For this review, take the finished solid that the model builds, in its own axes (mm). A direction names the side the tool comes from. Coordinates: 2 decimals unless noted, no trailing zeros. Write each loop counter-clockwise with the first axis right and the second up, starting at its lowest first coordinate (ties: lowest second). Pieces come first, ordered by that corner, then holes.
1) To check wall thickness, follow line 1 along Y through (x, z) = (-70.5, 8.9); line 2 along Y through (x, z) = (70.5, 4); line 3 along X through (y, z) = (-6, 2.5) (3 decimals). State the ranges of each line that lie inside material, in increasing order.
2) Insertion check: P1, Ø6.5, axis at x = 71.5, y = 67.5, coming from the -Z side; P2, Ø6.5, axis at x = -67.5, y = 66.5, coming from the -Z side; P3, Ø22, axis at x = -32.4, y = -6, coming from the +Z side. Each pin has a flat end and moves straight along its axis. Give the tip position at first contact, or say it passes through.
3) We need section B-B on y = -108. Write out the cut boundary in (x, z) (3 decimals).
4) We need section A-A on z = 3.75. Write out the cut boundary in (x, y) (3 decimals).
5) For faces 4 (the face through (-22.135, -5.548, 3.944)), 5 (the face through (-76.935, -132.852, 10.497)), 6 (the face through (90.5, -2, 6)), list the 3-axis set-ups (+Z, -Z, +X, -X, +Y, -Y) from which the entire face can be reached by the end or side of a thin tool; tool diameter is ignored.
6) Mouldability with a two-part tool opening along X and no side actions: class faces 1 (the face through (-88, 34, 12)), 2 (the face through (-90.5, -2, 6)), 3 (the face through (-35.5, -1.1, 9)) as pulls with the +X half, pulls with the -X half, needs draft (parallel to the pull), parting line crosses it, or undercut.
7) We need section C-C on x = -70.5. Write out the cut boundary in (y, z) (3 decimals).
from build123d import *

# Parameters (mm, degrees)
ESBO_O1_W                                           = 181
ESBO_O1_H                                           = 296
RESSALTO_EXTRUS_O1_DEPTH                            = 12
FILETE1_R                                           = 2
FILETE2_R                                           = 2
ESBO_O4_W                                           = 3.53
ESBO_O4_H                                           = 3.53
REBAIXO_PARA_PARAFUSO_COM_CABE_A_PANELA_D           = 7
REBAIXO_PARA_PARAFUSO_COM_CABE_A_PANELA_CBORE_D     = 13
REBAIXO_PARA_PARAFUSO_COM_CABE_A_PANELA_CBORE_DEPTH = 8
CORTE_EXTRUS_O1_REACH                               = 175.891
ESBO_O9_R                                           = 5.8
ESBO_O10_R                                          = 10.275
CORTE_EXTRUS_O2_DEPTH                               = 8
ESBO_O11_R                                          = 13.75
CORTE_EXTRUS_O3_DEPTH                               = 2
CORTE_EXTRUS_O4_DEPTH                               = 1.4
CORTE_EXTRUS_O5_DEPTH                               = 1.4


with BuildPart() as part:
    # Esboço1 → Ressalto-extrusão1 (new body)
    with BuildSketch(Plane.XY):
        Rectangle(ESBO_O1_W, ESBO_O1_H)
    extrude(amount=RESSALTO_EXTRUS_O1_DEPTH)

    # Filete1
    filete1_edges = [part.edges().sort_by_distance(p)[0] for p in [
        (-90.5, 148, 6),
    ]]
    fillet(filete1_edges, radius=FILETE1_R)

    # Filete2
    filete2_edges = [part.edges().sort_by_distance(p)[0] for p in [
        (90.5, -148, 6),
        (-90.5, -148, 6),
        (90.5, 148, 6),
    ]]
    fillet(filete2_edges, radius=FILETE2_R)

    # Varredura de corte1: sweep along a path in Esboço2
    with BuildLine(Plane.XY.offset(12)) as varredura_de_corte1_path:
        Line((-63.9, -140.1), (64.1, -140.1))
        ThreePointArc((64.1, -140.1), (78.242135624, -134.242135624), (84.1, -120.1))
        Line((84.1, -120.1), (84.1, 119.9))
        ThreePointArc((84.1, 119.9), (78.242135624, 134.042135624), (64.1, 139.9))
        Line((64.1, 139.9), (-63.9, 139.9))
        ThreePointArc((-63.9, 139.9), (-78.042135624, 134.042135624), (-83.9, 119.9))
        Line((-83.9, 119.9), (-83.9, -120.1))
        ThreePointArc((-83.9, -120.1), (-78.042135624, -134.242135624), (-63.9, -140.1))
    # Esboço4 → Varredura de corte1 (sweep, cut)
    with BuildSketch(Plane(origin=(0, 0, 0), x_dir=(1, 0, 0), z_dir=(0, 1, 0))):
        with Locations((-83.9, -10.8)):
            Rectangle(ESBO_O4_W, ESBO_O4_H)
    sweep(path=varredura_de_corte1_path.line, mode=Mode.SUBTRACT)

    # Rebaixo para parafuso com cabeça panela de M61 (through all)
    with Locations(Plane(origin=(0, 0, 0), x_dir=(-1, 0, 0), z_dir=(0, 0, -1))):
        with Locations((-70.5, 68), (70.5, 68), (70.5, -108), (-70.5, -108)):
            CounterBoreHole(REBAIXO_PARA_PARAFUSO_COM_CABE_A_PANELA_D / 2, REBAIXO_PARA_PARAFUSO_COM_CABE_A_PANELA_CBORE_D / 2, REBAIXO_PARA_PARAFUSO_COM_CABE_A_PANELA_CBORE_DEPTH)

    # Esboço9 → Corte-extrusão1 (cut, up to next)
    with BuildSketch(Plane(origin=(0, 0, 0), x_dir=(-1, 0, 0), z_dir=(0, 0, -1)), mode=Mode.PRIVATE) as corte_extrus_o1_sk1:
        with Locations((32.4, -6)):
            Circle(ESBO_O9_R)
    corte_extrus_o1_tool1 = extrude(corte_extrus_o1_sk1.sketch, amount=-CORTE_EXTRUS_O1_REACH, mode=Mode.PRIVATE) & part.part
    # Esboço9 → Corte-extrusão1 (cut, up to next)
    with BuildSketch(Plane(origin=(0, 0, 0), x_dir=(-1, 0, 0), z_dir=(0, 0, -1)), mode=Mode.PRIVATE) as corte_extrus_o1_sk2:
        with Locations((-32.4, 8.8)):
            Circle(ESBO_O9_R)
    corte_extrus_o1_tool2 = extrude(corte_extrus_o1_sk2.sketch, amount=-CORTE_EXTRUS_O1_REACH, mode=Mode.PRIVATE) & part.part
    add(corte_extrus_o1_tool1.solids().sort_by_distance((-32.4, -6, 0))[0], mode=Mode.SUBTRACT)
    add(corte_extrus_o1_tool2.solids().sort_by_distance((32.4, 8.8, 0))[0], mode=Mode.SUBTRACT)

    # Esboço10 → Corte-extrusão2 (cut)
    with BuildSketch(Plane(origin=(0, 0, 0), x_dir=(-1, 0, 0), z_dir=(0, 0, -1))):
        with Locations((32.4, -6)):
            Circle(ESBO_O10_R)
        with Locations((-32.4, 8.8)):
            Circle(ESBO_O10_R)
    extrude(amount=-CORTE_EXTRUS_O2_DEPTH, mode=Mode.SUBTRACT)

    # Esboço11 → Corte-extrusão3 (cut)
    with BuildSketch(Plane.XY.offset(12)):
        with Locations((32.4, 8.8)):
            Circle(ESBO_O11_R)
        with Locations((-32.4, -6)):
            Circle(ESBO_O11_R)
    extrude(amount=-CORTE_EXTRUS_O3_DEPTH, mode=Mode.SUBTRACT)

    # Esboço12 → Corte-extrusão4 (cut)
    with BuildSketch(Plane(origin=(0, 0, 0), x_dir=(-1, 0, 0), z_dir=(0, 0, -1))):
        with BuildLine():
            Line((-33.4, 19.075), (-33.4, 25.075))
            ThreePointArc((-33.4, 25.075), (-32.4, 26.075), (-31.4, 25.075))
            Line((-31.4, 25.075), (-31.4, 19.075))
            ThreePointArc((-31.4, 19.075), (-32.4, 18.075), (-33.4, 19.075))
        make_face()
    extrude(amount=-CORTE_EXTRUS_O4_DEPTH, mode=Mode.SUBTRACT)

    # Esboço13 → Corte-extrusão5 (cut)
    with BuildSketch(Plane(origin=(0, 0, 0), x_dir=(-1, 0, 0), z_dir=(0, 0, -1))):
        with BuildLine():
            Line((31.4, 4.275), (31.4, 9.275))
            ThreePointArc((31.4, 9.275), (32.4, 10.275), (33.4, 9.275))
            Line((33.4, 9.275), (33.4, 4.275))
            ThreePointArc((33.4, 4.275), (32.4, 3.275), (31.4, 4.275))
        make_face()
    extrude(amount=-CORTE_EXTRUS_O5_DEPTH, mode=Mode.SUBTRACT)


solid = part.part
Result:
1. line 1: y = -148 to -111.5, -104.5 to 64.5, 71.5 to 148
1. line 2: y = -148 to -114.5, -101.5 to 61.5, 74.5 to 148
1. line 3: x = -90.5 to -42.675, -22.125 to 90.5
2. P1: stops at z = 8
2. P2: stops at z = 0
2. P3: stops at z = 10
3. outline: (-90.5, 0) - (-77, 0) - (-77, 8) - (-74, 8) - (-74, 12) - (-82.135, 12) - (-82.135, 9.035) - (-85.665, 9.035) - (-85.665, 12) - (-90.5, 12) - close; (-67, 8) - (-64, 8) - (-64, 0) - (64, 0) - (64, 8) - (67, 8) - (67, 12) - (-67, 12) - close; (74, 8) - (77, 8) - (77, 0) - (90.5, 0) - (90.5, 12) - (85.865, 12) - (85.865, 9.035) - (82.335, 9.035) - (82.335, 12) - (74, 12) - close
4. outline: (-90.5, -146) arc R2 ccw to (-88.5, -148) - (88.5, -148) arc R2 ccw to (90.5, -146) - (90.5, 146) arc R2 ccw to (88.5, 148) - (-88.5, 148) arc R2 ccw to (-90.5, 146) - close; hole circle Ø13 at (-70.5, -108); hole circle Ø13 at (-70.5, 68); hole circle Ø20.55 at (-32.4, -6); hole circle Ø20.55 at (32.4, 8.8); hole circle Ø13 at (70.5, -108); hole circle Ø13 at (70.5, 68)
5. face 4: -Z
5. face 5: +Z
5. face 6: +Z, -Z, +X, +Y, -Y
6. face 1: needs draft
6. face 2: pulls with the -X half
6. face 3: undercut
7. outline: (-148, 0) - (-114.5, 0) - (-114.5, 8) - (-111.5, 8) - (-111.5, 12) - (-137.099, 12) - (-137.099, 9.035) - (-140.84, 9.035) - (-140.84, 12) - (-148, 12) - close; (-104.5, 8) - (-101.5, 8) - (-101.5, 0) - (61.5, 0) - (61.5, 8) - (64.5, 8) - (64.5, 12) - (-104.5, 12) - close; (71.5, 8) - (74.5, 8) - (74.5, 0) - (148, 0) - (148, 12) - (140.64, 12) - (140.64, 9.035) - (136.899, 9.035) - (136.899, 12) - (71.5, 12) - close
